```python
from build123d import *

# Parameters (mm, degrees)
SKETCH_1_W          = 112
SKETCH_1_H          = 66
SKETCH_1_R          = 1.5
SKETCH_1_R_2        = 2
SKETCH_1_R_3        = 11
SKETCH_1_R_4        = 5
EXTRUDE_1_DEPTH     = 3
FILLET_1_R          = 5
SKETCH_2_R          = 1.5
CUT_EXTRUDE_1_DEPTH = 10


with BuildPart() as part:
    # 草图1 → 凸台-拉伸1 (new body)
    with BuildSketch(Plane(origin=(0, 0, 0), x_dir=(1, 0, 0), z_dir=(0, 1, 0))):
        Rectangle(SKETCH_1_W, SKETCH_1_H)
        with Locations(Location((-50, 5, 0), (0, 0, 270))):
            Circle(SKETCH_1_R, mode=Mode.SUBTRACT)
        with Locations(Location((-50, -15, 0), (0, 0, 90))):
            Circle(SKETCH_1_R, mode=Mode.SUBTRACT)
        with Locations(Location((50, -15, 0), (0, 0, 270))):
            Circle(SKETCH_1_R, mode=Mode.SUBTRACT)
        with Locations(Location((50, 5, 0), (0, 0, 90))):
            Circle(SKETCH_1_R, mode=Mode.SUBTRACT)
        with Locations(Location((-14.5, 25.11473671, 0), (0, 0, 270))):
            Circle(SKETCH_1_R_2, mode=Mode.SUBTRACT)
        with Locations(Location((29, 0, 0), (0, 0, 270))):
            Circle(SKETCH_1_R_2, mode=Mode.SUBTRACT)
        with Locations(Location((-14.5, -25.11473671, 0), (0, 0, 270))):
            Circle(SKETCH_1_R_2, mode=Mode.SUBTRACT)
        with Locations(Location((0, 0, 0), (0, 0, 270))):
            Circle(SKETCH_1_R_3, mode=Mode.SUBTRACT)
        with Locations(Location((19.25, 0, 0), (0, 0, 270))):
            Circle(SKETCH_1_R_4, mode=Mode.SUBTRACT)
        with Locations(Location((-9.625, -16.670989023, 0), (0, 0, 270))):
            Circle(SKETCH_1_R_4, mode=Mode.SUBTRACT)
        with Locations(Location((-9.625, 16.670989023, 0), (0, 0, 270))):
            Circle(SKETCH_1_R_4, mode=Mode.SUBTRACT)
    extrude(amount=EXTRUDE_1_DEPTH)

    # 圆角1
    fillet_1_edges = [part.edges().sort_by_distance(p)[0] for p in [
        (56, 1.5, 33),
        (-56, 1.5, 33),
        (-56, 1.5, -33),
        (56, 1.5, -33),
    ]]
    fillet(fillet_1_edges, radius=FILLET_1_R)

    # 草图2 → 切除-拉伸1 (cut)
    with BuildSketch(Plane(origin=(0, 3, 0), x_dir=(1, 0, 0), z_dir=(0, 1, 0))):
        with Locations(Location((-48, 25, 0), (0, 0, 270))):
            Circle(SKETCH_2_R)
        with Locations(Location((-48, -25, 0), (0, 0, 270))):
            Circle(SKETCH_2_R)
        with Locations(Location((48, -25, 0), (0, 0, 270))):
            Circle(SKETCH_2_R)
        with Locations(Location((48, 25, 0), (0, 0, 270))):
            Circle(SKETCH_2_R)
    extrude(amount=-CUT_EXTRUDE_1_DEPTH, mode=Mode.SUBTRACT)


solid = part.part
```
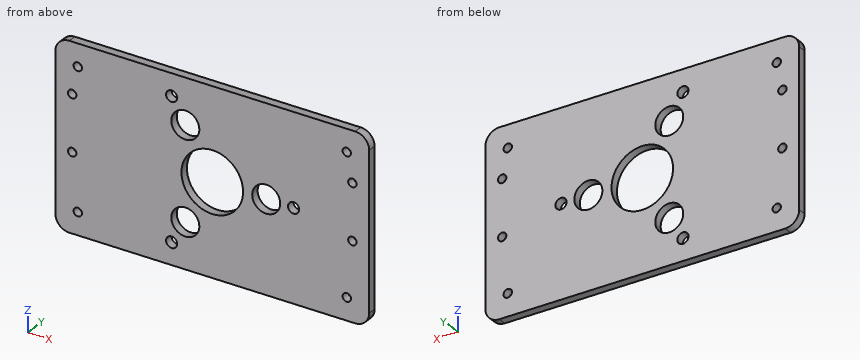
Input: part model. Units: mm. Frame: model coordinates. Coordinates: 2 decimals unless noted, no trailing zeros. Write each loop counter-clockwise with the first axis right and the second up, starting at its lowest first coordinate (ties: lowest second). Pieces come first, ordered by that corner, then holes.
1) Section B-B on z = 0. Output: boundary loops of the cut face in (x, y), and give its area (3 significant figures).
2) Section A-A on x = 19.25. Output: boundary loops of the cut face in (y, z).
3) Material intervals for line 1 along Z through (x, y) = (47.5, 0.5); line 2 along X through (y, z) = (2.75, 24); line 3 along X through (y, z) = (1.35, -1.5), sorted ascending.
4) Section D-D on z = 25. Output: boundary loops of the cut face in (x, y), and give its area (3 significant figures).
5) Section C-C on y = 1.1. State how many separate pieces and enclosed holes the cut face has, and give its area (3 significant figures).
6) Pin query (flat end, axial travel): pin 1 Ø3.5 at (x, z) = (-48, 25) entering from -Y. Return the tip coordinate at first contact, or that it passes through.
Check result:
1. outline: (-56, 0) - (-11, 0) - (-11, 3) - (-56, 3) - close; (11, 0) - (14.25, 0) - (14.25, 3) - (11, 3) - close; (24.25, 0) - (27, 0) - (27, 3) - (24.25, 3) - close; (31, 0) - (56, 0) - (56, 3) - (31, 3) - close
1. area: 228 mm2
2. outline: (0, -33) - (3, -33) - (3, -5) - (0, -5) - close; (0, 5) - (3, 5) - (3, 33) - (0, 33) - close
3. line 1: z = -33 to -26.41, -23.59 to 23.59, 26.41 to 33
3. line 2: x = -56 to -49.12, -46.88 to -16.16, -12.84 to 46.88, 49.12 to 56
3. line 3: x = -56 to -10.9, 10.9 to 14.48, 24.02 to 27.68, 30.32 to 56
4. outline: (-56, 0) - (-49.5, 0) - (-49.5, 3) - (-56, 3) - close; (-46.5, 0) - (-16.5, 0) - (-16.5, 3) - (-46.5, 3) - close; (-12.5, 0) - (46.5, 0) - (46.5, 3) - (-12.5, 3) - close; (49.5, 0) - (56, 0) - (56, 3) - (49.5, 3) - close
4. area: 306 mm2
5. separate pieces: 1
5. enclosed holes: 15
5. area: 6,660 mm2
6. pin 1: stops at y = 0
